Verification items for the finished model (mm, model axes). Face numbers are marked on the shaded views. A direction names the side the tool comes from. Give positions to 0.01 mm unless a question says otherwise; leave off trailing zeros. Loops run counter-clockwise (first coordinate to the right, second up) from the corner with the lowest first, then second, coordinate; pieces in that order, holes last. Notation, with made-up numbers: (10, 28.25) - (34, 28.25) arc R22 ccw to (34, 50.25) - close; hole circle Ø10 at (14, 85.5). An arc over 180 degrees is marked (long way). Answer in a Markdown table with one row per item.
```python
from build123d import *

# Parameters (mm, degrees)
BOSS_EXTRUDE1_DEPTH = 26
SKETCH2_R           = 8
CUT_EXTRUDE1_DEPTH  = 26
SKETCH3_R           = 9.5
SKETCH3_R_2         = 8
BOSS_EXTRUDE2_DEPTH = 3
BOSS_EXTRUDE4_DEPTH = 26
SKETCH5_R           = 1.55
CUT_EXTRUDE2_DEPTH  = 10.353024773
CUT_EXTRUDE3_DEPTH  = 27


with BuildPart() as part:
    # Sketch1 → Boss-Extrude1 (new body)
    with BuildSketch(Plane.XY):
        with BuildLine():
            Line((0, 0), (27, 0))
            Line((27, 0), (27, 26.5))
            Line((27, 26.5), (13.7, 26.5))
            Line((13.7, 26.5), (11.7, 26.5))
            Line((11.7, 26.5), (11.7, 24.839060942))
            ThreePointArc((11.7, 24.839060942), (12.011588642, 23.630402293), (12.868684584, 22.72302709))
            Line((12.868684584, 22.72302709), (13.7, 22.2))
            Line((13.7, 22.2), (13.7, 23.5))
            Line((13.7, 23.5), (24, 23.5))
            Line((24, 23.5), (24, 3))
            Line((24, 3), (0, 3))
            Line((0, 3), (0, 0))
        make_face()
    extrude(amount=BOSS_EXTRUDE1_DEPTH)

    # Sketch2 → Cut-Extrude1 (cut)
    with BuildSketch(Plane(origin=(27, 0, 0), x_dir=(0, 0, -1), z_dir=(1, 0, 0))):
        with Locations((-13, 13.25)):
            Circle(SKETCH2_R)
    extrude(amount=-CUT_EXTRUDE1_DEPTH, mode=Mode.SUBTRACT)

    # Sketch3 → Boss-Extrude2 (add)
    with BuildSketch(Plane(origin=(27, 0, 0), x_dir=(0, 0, -1), z_dir=(1, 0, 0))):
        with Locations((-13, 13.25)):
            Circle(SKETCH3_R)
        with Locations((-13, 13.25)):
            Circle(SKETCH3_R_2, mode=Mode.SUBTRACT)
    extrude(amount=BOSS_EXTRUDE2_DEPTH)

    # Sketch4 → Boss-Extrude4 (add)
    with BuildSketch(Plane(origin=(0, 0, 0), x_dir=(-1, 0, 0), z_dir=(0, 0, -1))):
        Polygon((-9.84807753, 3), (0, 3), (0, 4.736481777), align=None)
        Polygon((-27, 0), (0, 0), (-27, -4.760828479), align=None)
    extrude(amount=-BOSS_EXTRUDE4_DEPTH)

    # Sketch5 → Cut-Extrude2 (cut, through all)
    with BuildSketch(Plane(origin=(0.809986088, 4.593659375, 0), x_dir=(0.984807753, -0.173648178, 0), z_dir=(0.173648178, 0.984807753, 0))):
        with Locations((4.177518571, -5)):
            Circle(SKETCH5_R)
        with Locations((4.177518571, -21)):
            Circle(SKETCH5_R)
    extrude(amount=-CUT_EXTRUDE2_DEPTH, mode=Mode.SUBTRACT)

    # Sketch6 → Cut-Extrude3 (cut, through all)
    with BuildSketch(Plane(origin=(0, 0, 0), x_dir=(-1, 0, 0), z_dir=(0, 0, -1))):
        Polygon((0, 0), (-0.809986088, 4.593659375), (0, 4.736481777), align=None)
    extrude(amount=-CUT_EXTRUDE3_DEPTH, mode=Mode.SUBTRACT)


solid = part.part
```
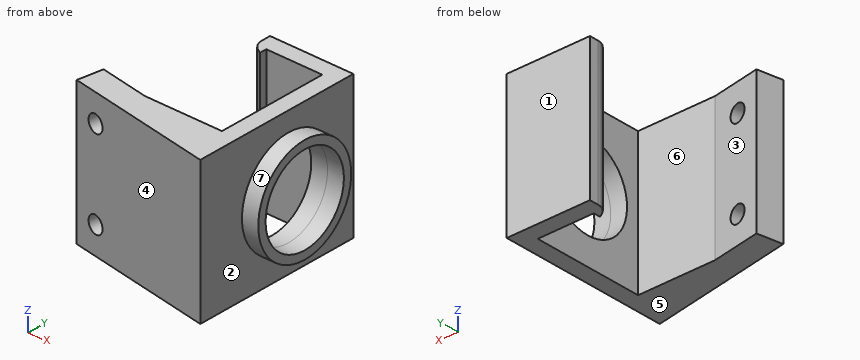
Q1. Go/stop test with flat-tipped pins: P1, Ø10, axis at y = 7, z = 4.5, coming from the -X side; P2, Ø1, axis at y = 23, z = 10.5, coming from the +X side; P3, Ø10, axis at x = 15.5, z = 11.5, coming from the -Y side; P4, Ø6, axis at x = 26.5, y = -1, coming from the -Z side. Record where each tip stops, or that it passes through.
Completed:
| item | result |
|---|---|
| P1 | x = 0.35 |
| P2 | x = 27 |
| P3 | y = -3.61 |
| P4 | z = 0 |
Q2. Sectioned sample at A-A (y = 13.25). Record the cut outline in (x, z).
Completed:
| item | result |
|---|---|
| outline | (24, 0) - (27, 0) - (27, 3.5) - (30, 3.5) - (30, 5) - (24, 5) - close; (24, 21) - (30, 21) - (30, 22.5) - (27, 22.5) - (27, 26) - (24, 26) - close |
Q3. Sectioned sample at D-D (x = 28.25). Record the cut outline in (y, z), and give its area (3 significant figures).
Completed:
| item | result |
|---|---|
| outline | circle Ø19 at (13.25, 13); hole circle Ø16 at (13.25, 13) |
| area | 82.5 mm^2 |
Q4. Sectioned sample at C-C (z = 20). Record the cut outline in (x, y).
Completed:
| item | result |
|---|---|
| outline | (0, 0) - (2.95, -0.52) - (3.76, 4.07) - (0.81, 4.59) - close; (5.28, -0.93) - (27, -4.76) - (27, 6.83) - (30, 6.83) - (30, 9.38) - (24, 9.38) - (24, 3) - (9.85, 3) - (6.09, 3.66) - close; (11.7, 24.84) arc R2.5 ccw to (12.87, 22.72) - (13.7, 22.2) - (13.7, 23.5) - (24, 23.5) - (24, 17.12) - (30, 17.12) - (30, 19.67) - (27, 19.67) - (27, 26.5) - (11.7, 26.5) - close |
Q5. Thickness scan on line 1 (Y direction, x = 28.5, z = 13); line 2 (Z direction, x = 4.25, y = 3.5); line 3 (Y direction, x = 23.75, z = 5.75). Record the ranges inside material, lowest first.
Completed:
| item | result |
|---|---|
| line 1 | 3.75 to 5.25, 21.25 to 22.75 |
| line 2 | 0 to 3.57, 6.43 to 19.57, 22.43 to 26 |
| line 3 | -4.19 to 3, 23.5 to 26.5 |
Q6. Tool access check on the marked faces 5, 6 and 7. Record the directions out of +Z, -Z, +X, -X, +Y, -Y that give a thin tool (end or side, any length) a straight path to the whole face; none if there is none.
Completed:
| item | result |
|---|---|
| face 5 | -Z, +X, -X, +Y, -Y |
| face 6 | +Z, -Z |
| face 7 | +X |
Q7. Draft check along X on the marked faces 1, 2, 3 and 4. Enter one of: +X half, -X half, draft (parallel to the pull), parting line (faces both ways), or undercut.
Completed:
| item | result |
|---|---|
| face 1 | draft |
| face 2 | +X half |
| face 3 | undercut |
| face 4 | -X half |
Q8. Sectioned sample at B-B (z = 13). Record the cut outline in (x, y), and give its area (3 significant figures).
Completed:
| item | result |
|---|---|
| outline | (0, 0) - (27, -4.76) - (27, 3.75) - (30, 3.75) - (30, 5.25) - (24, 5.25) - (24, 3) - (9.85, 3) - (0.81, 4.59) - close; (11.7, 24.84) arc R2.5 ccw to (12.87, 22.72) - (13.7, 22.2) - (13.7, 23.5) - (24, 23.5) - (24, 21.25) - (30, 21.25) - (30, 22.75) - (27, 22.75) - (27, 26.5) - (11.7, 26.5) - close |
| area | 221 mm^2 |
